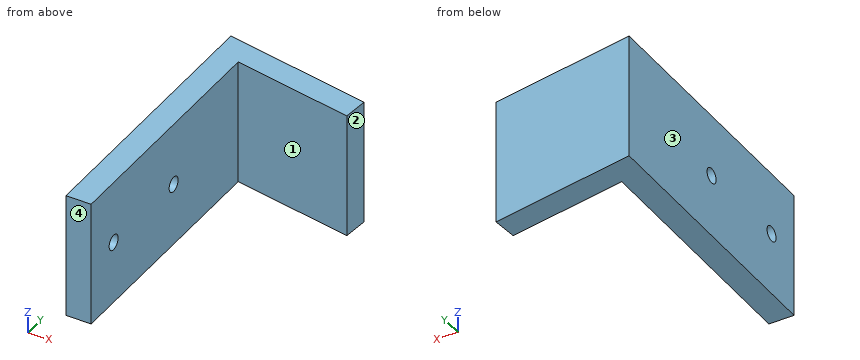
```python
from build123d import *

# Parameters (mm, degrees)
BOSS_EXTRU_1_DEPTH      = 50
ESQUISSE2_R             = 3
ENL_V_MAT_EXTRU_1_DEPTH = 10


with BuildPart() as part:
    # Esquisse1 → Boss.-Extru.1 (new body)
    with BuildSketch(Plane.XY):
        Polygon((0, 0), (0, -110), (10, -110), (10, -11.917535926), (58.206757919, -20.417687999), (59.088465181, -10.41889066), align=None)
    extrude(amount=BOSS_EXTRU_1_DEPTH)

    # Esquisse2 → Enlèv. mat.-Extru.1 (cut)
    with BuildSketch(Plane.ZY):
        with Locations(Location((25, -95, 0), (0, 0, 270))):
            Circle(ESQUISSE2_R)
        with Locations(Location((25, -55, 0), (0, 0, 270))):
            Circle(ESQUISSE2_R)
    extrude(amount=-ENL_V_MAT_EXTRU_1_DEPTH, mode=Mode.SUBTRACT)


solid = part.part
```
Verification items for the finished model (mm, model axes). Face numbers are marked on the shaded views. Give positions to 0.01 mm unless a question says otherwise; leave off trailing zeros. Order: outer loops, then holes, each group sorted by start corner. A loop starts at its lowest first (then second) coordinate and runs counter-clockwise, first axis right, second up. Notation, with made-up numbers: (69.5, 19.25) - (124.5, 19.25) arc R22 ccw to (124.5, 35.25) - close; hole circle Ø2 at (70.5, 45.25). An arc over 180 degrees is marked (long way). Answer as CSV lines item,"result". Start each with the question number.
Item 1: Section check C-C, the plane z = 41. Record the boundary of the cut face in (x, y), plus the area to 3 significant figures.
Item 2: Material ranges on L1, parallel to Z at x = 3, y = -55; L2, parallel to X at y = -91.5, z = 12; L3, parallel to Y at x = 45, z = 25.5, recorded low to high.
Item 3: Mould release check, pull along X, two halves, no side actions. Record for the marked faces 1, 2, 3 and 4: released by +X, released by -X, zero draft, split by the parting line, or undercut.
Item 4: Section check A-A, the plane z = 25. Record the boundary of the cut face in (x, y).
Item 5: Section check D-D, the plane x = 24. Record the boundary of the cut face in (y, z), plus the area to 3 significant figures.
Item 6: Gauge pin test, flat ends, axial feed: pin 1 (12 mm diameter, centred on y = -57.5, z = 25, fed in from -X); pin 2 (3 mm diameter, centred on y = -18.5, z = 6.5, fed in from +X); pin 3 (4 mm diameter, centred on y = -34.5, z = 26, fed in from +X); pin 4 (12 mm diameter, centred on y = -21.5, z = 21.5, fed in from +X). Record the tip position at first contact, or that the pin passes through.
Item 7: Section check B-B, the plane y = -95. Record the boundary of the cut face in (x, z), plus the area to 3 significant figures.
Filled in:
1,outline,"(0, -110) - (10, -110) - (10, -11.92) - (58.21, -20.42) - (59.09, -10.42) - (0, 0) - close"
1,area,"1,590 mm^2"
2,L1,"0 to 22, 28 to 50"
2,L2,"0 to 10"
2,L3,"-18.09 to -7.93"
3,face 1,"undercut"
3,face 2,"released by +X"
3,face 3,"released by -X"
3,face 4,"zero draft"
4,outline,"(0, -110) - (10, -110) - (10, -98) - (0, -98) - close; (0, -92) - (10, -92) - (10, -58) - (0, -58) - close; (0, -52) - (10, -52) - (10, -11.92) - (58.21, -20.42) - (59.09, -10.42) - (0, 0) - close"
5,outline,"(-14.39, 0) - (-4.23, 0) - (-4.23, 50) - (-14.39, 50) - close"
5,area,"508 mm^2"
6,pin 1,"x = 0"
6,pin 2,"x = 58.51"
6,pin 3,"x = 10"
6,pin 4,"x = 58.64"
7,outline,"(0, 0) - (10, 0) - (10, 22) - (0, 22) - close; (0, 28) - (10, 28) - (10, 50) - (0, 50) - close"
7,area,"440 mm^2"
